from build123d import *

# Parameters (mm, degrees)
SKETCH_W        = 6
SKETCH_H        = 25
PAD_DEPTH       = 2
SKETCH001_W     = 6
SKETCH001_H     = 3
PAD001_DEPTH    = 10
FILLET_R        = 2
SKETCH002_R     = 1.1
POCKET_DEPTH    = 5
SKETCH003_R     = 1.65
POCKET001_DEPTH = 5


with BuildPart() as part:
    # Sketch → Pad (new body)
    with BuildSketch(Plane.XY):
        with Locations((3, 12.5)):
            Rectangle(SKETCH_W, SKETCH_H)
    extrude(amount=PAD_DEPTH)

    # Sketch001 (on Face6 of Pad) → Pad001 (join)
    with BuildSketch(Plane.XY.offset(2)):
        with Locations((3, 1.5)):
            Rectangle(SKETCH001_W, SKETCH001_H)
    extrude(amount=PAD001_DEPTH)

    # Fillet
    fillet_edges = [part.edges().sort_by_distance(p)[0] for p in [
        (3, 3, 2),
    ]]
    fillet(fillet_edges, radius=FILLET_R)

    # Sketch002 (on Face2 of Fillet) → Pocket (cut)
    with BuildSketch(Plane.XY.offset(2)):
        with Locations((3, 23.17265)):
            Circle(SKETCH002_R)
        with Locations((3, 7.17265)):
            Circle(SKETCH002_R)
    extrude(amount=-POCKET_DEPTH, mode=Mode.SUBTRACT)

    # Sketch003 (on Face13 of Pocket) → Pocket001 (cut)
    with BuildSketch(Plane.XZ):
        with Locations((3, 7)):
            Circle(SKETCH003_R)
    extrude(amount=-POCKET001_DEPTH, mode=Mode.SUBTRACT)


solid = part.part
Geometry: final body of the model. Coordinates: model frame, mm. A direction names the side the tool comes from. Give positions to 0.01 mm unless a question says otherwise; leave off trailing zeros. Loops run counter-clockwise (first coordinate to the right, second up) from the corner with the lowest first, then second, coordinate; pieces in that order, holes last. Notation, with made-up numbers: M 65,55.5 L 120,55.5 A30 ccw 120,89.5 Z; hole C 12.5,-24.75 d1. An arc over 180 degrees is marked long. Put each result on its own line as item: value. Start each with the question number.
1) Pull-direction query (X, two-part tool) for faces 3 (the flat face through (6, 9, 1)), 4 (the flat face through (3, 0, 5)), 5 (the cylindrical face through (4.016, 6.751, 1.014)); classes: pulls with the +X half, pulls with the -X half, needs draft (parallel to the pull), parting line crosses it, or undercut.
2) Cut plane B-B (x = 3). Output: boundary loops of the cut face in (y, z), then the cut area to 3 significant figures.
3) Ray query, line 1 along Y through (x, z) = (3, 0.95); line 2 along Z through (x, y) = (3, 1.6); line 3 along Y through (x, z) = (0.8, 7.5). Return the intervals inside material, ascending.
4) Cut plane A-A (z = 7). Output: boundary loops of the cut face in (x, y).
5) Cut plane D-D (x = 0.6). Output: boundary loops of the cut face in (y, z).
6) Access query for faces 1 (the flat face through (3, 3, 9)), 2 (the cylindrical face through (2.6, 1.5, 5.4)). Directions: +Z, -Z, +X, -X, +Y, -Y. A direction counts if a zero-diameter tool reaches every point of the face in a straight line with its end or side. Return the directions, or none.
7) Contact query for a flat-ended pin moving along its axis: pin 1 (2.5 mm diameter, centred on x = 3, y = 23.17, fed in from -Z). Output: stop coordinate, or through.
8) Cut plane C-C (y = 12.25). Output: boundary loops of the cut face in (x, z).
Verdict:
1. face 3: pulls with the +X half
1. face 4: needs draft
1. face 5: undercut
2. outline: M 0,0 L 6.07,0 L 6.07,2 L 5,2 A2 cw 3,4 L 3,5.35 L 0,5.35 Z; M 0,8.65 L 3,8.65 L 3,12 L 0,12 Z; M 8.27,0 L 22.07,0 L 22.07,2 L 8.27,2 Z; M 24.27,0 L 25,0 L 25,2 L 24.27,2 Z
2. area: 62.2 mm2
3. line 1: 0 to 6.07, 8.27 to 22.07, 24.27 to 25
3. line 2: 0 to 5.35, 8.65 to 12
3. line 3: 0 to 3
4. outline: M 0,0 L 1.35,0 L 1.35,3 L 0,3 Z; M 4.65,0 L 6,0 L 6,3 L 4.65,3 Z
5. outline: M 0,0 L 25,0 L 25,2 L 5,2 A2 cw 3,4 L 3,12 L 0,12 Z
6. face 1: +Z, +X, -X, +Y
6. face 2: +Y, -Y
7. pin 1: z = 0
8. outline: M 0,0 L 6,0 L 6,2 L 0,2 Z
